Study the drawing (mm; zero at the part's minimum x, y, z) and answer. Give positions to 0.01 mm unless a question says otherwise; leave off trailing zeros. Write each loop counter-clockwise with the first axis right and the second up, starting at its lowest first coordinate (ties: lowest second). Pieces come first, ordered by that corner, then holes.
1) Straight lines are drawn through the part: probe 1 along Y at (x, z) = (5, 45.72) (1 decimal); probe 2 along Y at (x, z) = (7.75, 47.5) (1 decimal); probe 3 along Y at (x, z) = (8.75, 42). For each, find the intervals that lie inside material, in ascending order.
2) Find section B-B (y = 45.72). Determine the outline of the cut face in (x, z) (1 decimal).
3) Determine the mould class of the marked faces 1, 2 and 3 for opening direction Y: pulls with the +Y half, pulls with the -Y half, needs draft (parallel to the pull), parting line crosses it, or undercut.
4) Find section C-C (z = 58.5). Determine the outline of the cut face in (x, y) (1 decimal).
5) Find section A-A (z = 45.72). Determine the outline of the cut face in (x, y) (1 decimal).
6) Given pin 1 Ø17 at (y, z) = (45.72, 45.72) entering from +X; pin 2 Ø4 at (x, y) = (6.5, 42.5) entering from +Z; pin 3 Ø1.5 at (x, y) = (7, 12) entering from -Z (1 decimal); pin 4 Ø1 at (x, z) = (6.5, 44.5) entering from -Y, each flat-ended and moving along its own axis, determine where each tip first touches the part or whether it passes through.
7) Find section D-D (x = 8.25). Determine the outline of the cut face in (y, z) (1 decimal).
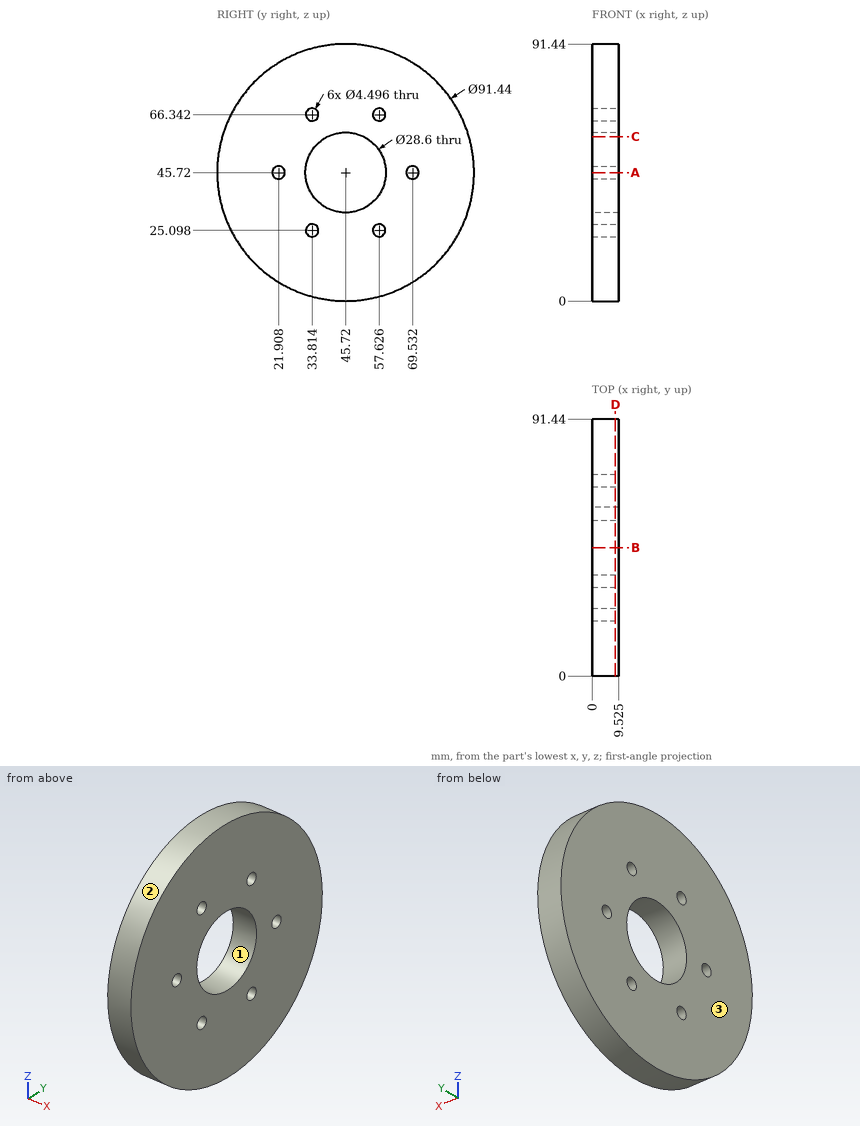
Results:
1. probe 1: y = 0 to 19.7, 24.2 to 31.4, 60 to 67.3, 71.8 to 91.4
1. probe 2: y = 0 to 20.5, 23.3 to 31.5, 59.9 to 68.2, 70.9 to 91.4
1. probe 3: y = 0.15 to 31.91, 59.53 to 91.29
2. outline: (0, 0) - (9.5, 0) - (9.5, 31.4) - (0, 31.4) - close; (0, 60) - (9.5, 60) - (9.5, 91.4) - (0, 91.4) - close
3. face 1: undercut
3. face 2: parting line crosses it
3. face 3: needs draft
4. outline: (0, 1.8) - (9.5, 1.8) - (9.5, 39.3) - (0, 39.3) - close; (0, 52.1) - (9.5, 52.1) - (9.5, 89.6) - (0, 89.6) - close
5. outline: (0, 0) - (9.5, 0) - (9.5, 19.7) - (0, 19.7) - close; (0, 24.2) - (9.5, 24.2) - (9.5, 31.4) - (0, 31.4) - close; (0, 60) - (9.5, 60) - (9.5, 67.3) - (0, 67.3) - close; (0, 71.8) - (9.5, 71.8) - (9.5, 91.4) - (0, 91.4) - close
6. pin 1: passes through
6. pin 2: stops at z = 91.42
6. pin 3: stops at z = 14
6. pin 4: stops at y = 0.01
7. outline: circle Ø91.4 at (45.7, 45.7); hole circle Ø4.5 at (21.9, 45.7); hole circle Ø28.6 at (45.7, 45.7); hole circle Ø4.5 at (33.8, 25.1); hole circle Ø4.5 at (33.8, 66.3); hole circle Ø4.5 at (57.6, 25.1); hole circle Ø4.5 at (57.6, 66.3); hole circle Ø4.5 at (69.5, 45.7)
